Input: dimensioned drawing with shaded views. Units: mm. Origin: part minimum x, y, z. A direction names the side the tool comes from. Round coordinates to 2 decimals unless told otherwise and drop trailing zeros. Loops run counter-clockwise (first coordinate to the right, second up) from the corner with the lowest first, then second, coordinate; pieces in that order, holes last. Notation, with made-up numbers: (82, 48.25) - (111, 48.25) arc R24 cw to (111, 74.25) - close; hole circle Ø9 at (11, 9.5). An arc over 180 degrees is marked (long way). Write each question's results on one line, items separated by ' | '.
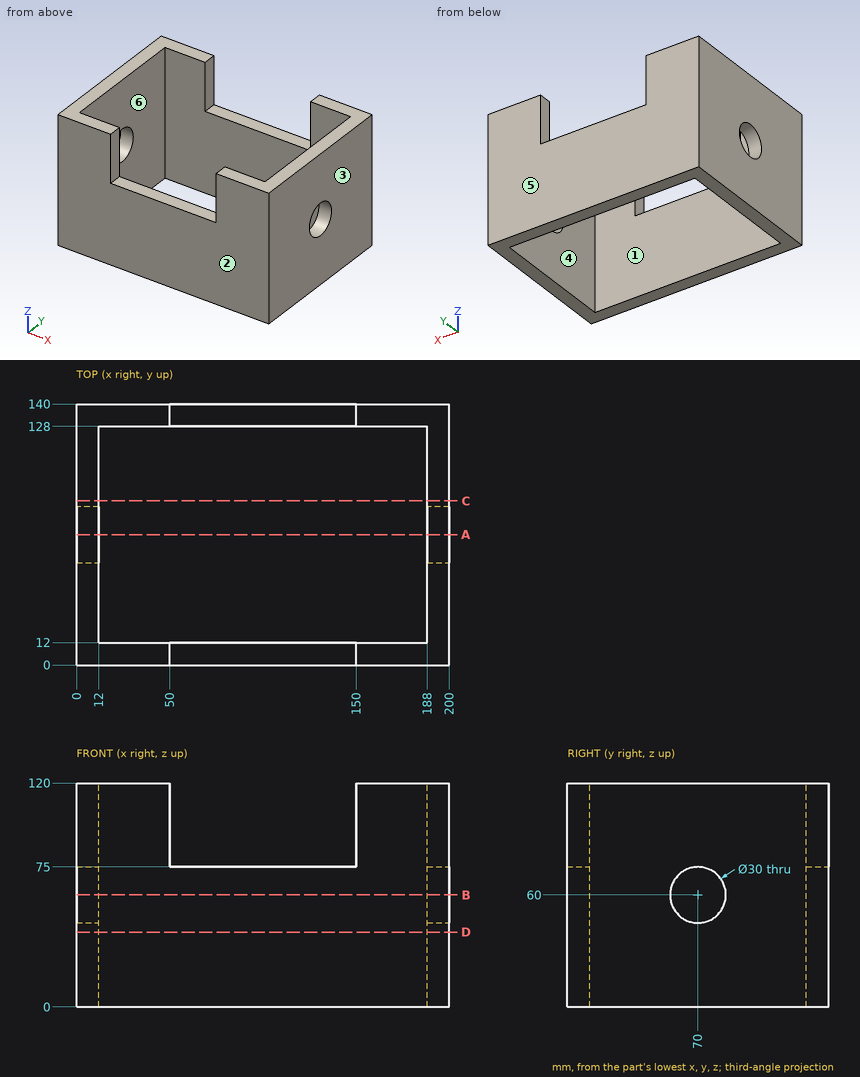
1. Set-up query: the marked faces 1 and 2. Return all of +Z, -Z, +X, -X, +Y, -Y with unobstructed straight access to the full face (end or side cutting, diameter ignored); none if empty.
Answer:
face 1: +Z, -Z | face 2: +Z, -Z, +X, -X, -Y
2. Section query D-D, the plane z = 40. Output: boundary loops of the cut face in (x, y).
Answer:
outline: (0, 0) - (200, 0) - (200, 140) - (0, 140) - close; hole (12, 12) - (188, 12) - (188, 128) - (12, 128) - close
3. Mould query, pull axis X, two halves, no side actions, for the marked faces 3, 4, 5 and 6. Classes: pulls with the +X half, pulls with the -X half, needs draft (parallel to the pull), parting line crosses it, or undercut.
Answer:
face 3: pulls with the +X half | face 4: undercut | face 5: needs draft | face 6: undercut
4. Section query B-B, the plane z = 60. Output: boundary loops of the cut face in (x, y), plus the area to 3 significant figures.
Answer:
outline: (0, 0) - (200, 0) - (200, 55) - (188, 55) - (188, 12) - (12, 12) - (12, 55) - (0, 55) - close; (0, 85) - (12, 85) - (12, 128) - (188, 128) - (188, 85) - (200, 85) - (200, 140) - (0, 140) - close | area: 6,860 mm^2
5. Section query C-C, the plane y = 88. Output: boundary loops of the cut face in (x, z).
Answer:
outline: (0, 0) - (12, 0) - (12, 120) - (0, 120) - close; (188, 0) - (200, 0) - (200, 120) - (188, 120) - close
6. Contact query for flat-ended pins moving along their axis: pin 1 (10 mm diameter, centred on x = 60, y = 123.5, fed in from +Z); pin 2 (12 mm diameter, centred on y = 72, z = 55, fed in from -X). Output: stop coordinate, or through.
Answer:
pin 1: z = 75 | pin 2: through
7. Line query: line 1 (Y direction, x = 111, z = 7); line 2 (X direction, y = 132, z = 95.5); line 3 (Z direction, x = 197, y = 70). Output: solid intervals per line, ascending. Write a range as [from, to].
Answer:
line 1: [0, 12], [128, 140] | line 2: [0, 50], [150, 200] | line 3: [0, 45], [75, 120]
8. Section query A-A, the plane y = 70. Output: boundary loops of the cut face in (x, z).
Answer:
outline: (0, 0) - (12, 0) - (12, 45) - (0, 45) - close; (0, 75) - (12, 75) - (12, 120) - (0, 120) - close; (188, 0) - (200, 0) - (200, 45) - (188, 45) - close; (188, 75) - (200, 75) - (200, 120) - (188, 120) - close
